Source: CAD feature listing. Evaluate the final solid. Frame: model axes, mm. A direction names the side the tool comes from. Round coordinates to 2 decimals unless told otherwise and drop trailing zeros. Write each loop counter-clockwise with the first axis right and the second up, starting at its lowest first coordinate (ties: lowest second). Pieces come first, ordered by that corner, then holes.
```python
from build123d import *

# Parameters (mm, degrees)
SKETCH1_R           = 1.65
SKETCH1_W           = 30.68
SKETCH1_H           = 2.7
SKETCH1_W_2         = 15.28
BOSS_EXTRUDE1_DEPTH = 2.7


with BuildPart() as part:
    # Sketch1 → Boss-Extrude1 (new body)
    with BuildSketch(Plane(origin=(0, 0, 0), x_dir=(1, 0, 0), z_dir=(0, 1, 0))):
        with BuildLine():
            Line((-46, 0), (46, 0))
            ThreePointArc((46, 0), (62.780941571, 3.32568378), (77.025151087, 12.8))
            Line((77.025151087, 12.8), (46.015151087, 12.8))
            Line((46.015151087, 12.8), (46.015151087, 15.5))
            Line((46.015151087, 15.5), (73.995151087, 15.5))
            Line((73.995151087, 15.5), (73.995151087, 35.5))
            Line((73.995151087, 35.5), (38.2, 35.5))
            Line((38.2, 35.5), (38.2, 65.5))
            Line((38.2, 65.5), (-38.2, 65.5))
            Line((-38.2, 65.5), (-38.2, 35.5))
            Line((-38.2, 35.5), (-73.995151087, 35.5))
            Line((-73.995151087, 35.5), (-73.995151087, 15.5))
            Line((-73.995151087, 15.5), (-46.015151087, 15.5))
            Line((-46.015151087, 15.5), (-46.015151087, 12.8))
            Line((-46.015151087, 12.8), (-77.025151087, 12.8))
            ThreePointArc((-77.025151087, 12.8), (-62.780941571, 3.32568378), (-46, 0))
        make_face()
        with Locations((46, 28.5)):
            Circle(SKETCH1_R, mode=Mode.SUBTRACT)
        with Locations((46, 7)):
            Circle(SKETCH1_R, mode=Mode.SUBTRACT)
        with Locations((-46, 7)):
            Circle(SKETCH1_R, mode=Mode.SUBTRACT)
        with Locations((-46, 28.5)):
            Circle(SKETCH1_R, mode=Mode.SUBTRACT)
        with Locations((0, 14.15)):
            Rectangle(SKETCH1_W, SKETCH1_H, mode=Mode.SUBTRACT)
        with Locations((-15.28, 61.45)):
            Rectangle(SKETCH1_W_2, SKETCH1_H, mode=Mode.SUBTRACT)
        with Locations((15.28, 61.45)):
            Rectangle(SKETCH1_W_2, SKETCH1_H, mode=Mode.SUBTRACT)
    extrude(amount=BOSS_EXTRUDE1_DEPTH)


solid = part.part
```
Q1. Section query B-B, the plane y = 1.9. Give the number of separate pieces and of enclosed holes in the cut face, and give its area (3 significant figures).
Q2. Mould query, pull axis X, two halves, no side actions, for faces 1 (the face through (62.558, 1.331, -3.234)), 2 (the face through (15, 1, -62.8)), 3 (the face through (60, 1, -15.5)). Classes: pulls with the +X half, pulls with the -X half, needs draft (parallel to the pull), parting line crosses it, or undercut.
Q3. Section query C-C, the plane x = -67. Output: boundary loops of the cut face in (y, z).
Q4. Set-up query: faces 4 (the face through (62, 1, -12.8)), 5 (the face through (38.2, 1, -50)), 6 (the face through (-60, 1, -15.5)), 7 (the face through (22.92, 1, -61)), 8 (the face through (-56, 1, -35.5)). Return all of +Z, -Z, +X, -X, +Y, -Y with unobstructed straight access to the full face (end or side cutting, diameter ignored); none if empty.
Q5. Section query D-D, the plane z = -7. Output: boundary loops of the cut face in (x, y), and give its area (3 significant figures).
Q6. Pin query (flat end, axial travel): P1, Ø1.3, axis at y = 1, z = -14, coming from the -X side; P2, Ø0.8, axis at y = 1, z = -13.5, coming from the +X side; P3, Ø0.8, axis at y = 0.5, z = -61.5, coming from the -X side. Return the tip coordinate at first contact, or that it passes through.
Q7. Section query A-A, the plane z = -28.5. Output: boundary loops of the cut face in (x, y).
Q8. Line query: line 1 (X direction, y = 1.25, z = -28.5); line 2 (Z direction, x = -9.5, y = 1.8); line 3 (X direction, y = 1.65, z = -7). Output: solid intervals per line, ascending.
Filled in:
1. separate pieces: 1
1. enclosed holes: 7
1. area: 7,030 mm2
2. face 1: pulls with the +X half
2. face 2: undercut
2. face 3: needs draft
3. outline: (0, -35.5) - (2.7, -35.5) - (2.7, -15.5) - (0, -15.5) - close; (0, -12.8) - (2.7, -12.8) - (2.7, -5.33) - (0, -5.33) - close
4. face 4: +X, +Y, -Y
4. face 5: -Z, +X, +Y, -Y
4. face 6: -X, +Y, -Y
4. face 7: +Y, -Y
4. face 8: -Z, -X, +Y, -Y
5. outline: (-69.81, 0) - (-47.65, 0) - (-47.65, 2.7) - (-69.81, 2.7) - close; (-44.35, 0) - (44.35, 0) - (44.35, 2.7) - (-44.35, 2.7) - close; (47.65, 0) - (69.81, 0) - (69.81, 2.7) - (47.65, 2.7) - close
5. area: 359 mm2
6. P1: stops at x = -46.02
6. P2: stops at x = 46.02
6. P3: stops at x = -38.2
7. outline: (-74, 0) - (-47.65, 0) - (-47.65, 2.7) - (-74, 2.7) - close; (-44.35, 0) - (44.35, 0) - (44.35, 2.7) - (-44.35, 2.7) - close; (47.65, 0) - (74, 0) - (74, 2.7) - (47.65, 2.7) - close
8. line 1: x = -74 to -47.65, -44.35 to 44.35, 47.65 to 74
8. line 2: z = -65.5 to -62.8, -60.1 to -15.5, -12.8 to 0
8. line 3: x = -69.81 to -47.65, -44.35 to 44.35, 47.65 to 69.81
